Build history of the part. All positions in model axes, mm. Face numbers are marked on the shaded views. A direction names the side the tool comes from. Coordinates: 2 decimals unless noted, no trailing zeros. Loops run counter-clockwise (first coordinate to the right, second up) from the corner with the lowest first, then second, coordinate; pieces in that order, holes last. Notation, with made-up numbers: (20, 67) - (35, 67) arc R25 ccw to (35, 92) - close; hole circle Ø3 at (-9.5, -22). An arc over 180 degrees is marked (long way). One line per item, written item: value.
Autodesk Inventor part; units mm, degrees
ref_plane "YZ Plane" through (0, 0, 0) normal (1, 0, 0) x (0, 1, 0)
ref_plane "XZ Plane" through (0, 0, 0) normal (0, 1, 0) x (-1, 0, 0)
ref_plane "XY Plane" through (0, 0, 0) normal (0, 0, 1) x (1, 0, 0)
sketch "Sketch1" plane through (0, 0, 0) normal (0, 1, 0) x (-1, 0, 0)
  circle A0 centre (0, 0) radius 3.2
  dimension "d0" = 6.4
extrude "Extrusion1" add sketch "Sketch1" against normal blind 42
sketch "Sketch2" plane through (0, -42, 0) normal (0, -1, 0) x (1, 0, 0)
  circle A0 centre (0, 0) radius 6.5
  dimension "d3" = 13
extrude "Extrusion2" add sketch "Sketch2" against normal blind 20
sketch "Sketch3" plane through (0, 0, 0) normal (0, 1, 0) x (1, 0, 0)
  circle A0 centre (0, 0) radius 3.2
  line L0 (0, -3.2) -> (0, 3.2) construction
  circle A1 centre (0, -1.2) radius 0.5
  circle A2 centre (0, 1.4) radius 0.5
  dimension "d6" = 0
  dimension "d7" = 1
  dimension "d8" = 1
  dimension "d9" = 1.8
  dimension "d10" = 2.6
extrude "Extrusion3" add sketch "Sketch3" along normal blind 6 contours A1 | A2
fillet "Fillet1" radius 0.5 2 edges at (-0.5, 6, -1.4) (-0.5, 6, 1.2)
properties part number "Arc Water Sensor"
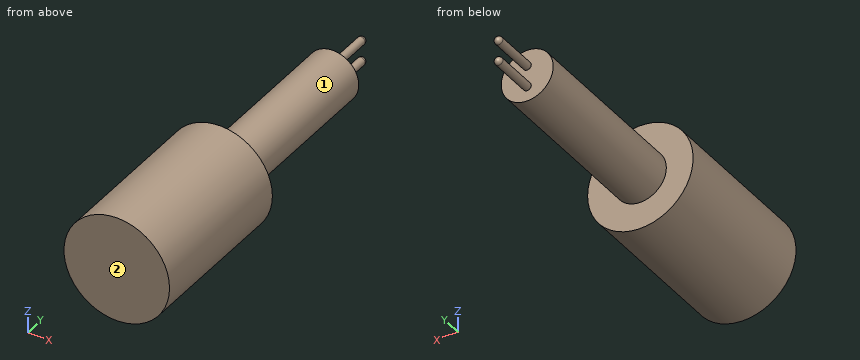
Item 1: Probe probe 1 along Y at (x, z) = (3.5, -0.25); probe 2 along Y at (x, z) = (-2.75, -0.5); probe 3 along Z at (x, y) = (-0.25, -15). List the from-to ranges inside material, lowest first. Write a range as from..to.
Check result:
probe 1: y = -42..-22
probe 2: y = -42..0
probe 3: z = -3.19..3.19
Item 2: Cut at C-C, the plane y = -11.5. Write the cut outline in (x, z).
Check result:
outline: circle Ø6.4 at (0, 0)
Item 3: Cut at B-B, the plane z = -1.4. Write the cut outline in (x, y).
Check result:
outline: (-6.35, -42) - (6.35, -42) - (6.35, -22) - (2.88, -22) - (2.88, 0) - (0.5, 0) - (0.5, 5.5) arc R0.5 ccw to (-0.5, 5.5) - (-0.5, 0) - (-2.88, 0) - (-2.88, -22) - (-6.35, -22) - close
Item 4: Cut at A-A, the plane x = 0. Write the cut outline in (y, z).
Check result:
outline: (-42, -6.5) - (-22, -6.5) - (-22, -3.2) - (0, -3.2) - (0, -1.9) - (5.5, -1.9) arc R0.5 ccw to (5.5, -0.9) - (0, -0.9) - (0, 0.7) - (5.5, 0.7) arc R0.5 ccw to (5.5, 1.7) - (0, 1.7) - (0, 3.2) - (-22, 3.2) - (-22, 6.5) - (-42, 6.5) - close
Item 5: Drop flat-ended pins along their axis: P1, Ø1, axis at x = 1.5, y = -21, coming from the -Z side; P2, Ø5, axis at x = -5, y = -12.5, coming from the -Z side; P3, Ø6, axis at x = 4, z = -3.5, coming from the +Y side. Give the stop position or say it passes through.
Check result:
P1: stops at z = -3.04
P2: stops at z = -2
P3: stops at y = 0
Item 6: Tool access for the marked faces 1 and 2: list every direction of +Z, -Z, +X, -X, +Y, -Y with a clear straight run to the whole face (end or side of a thin tool).
Check result:
face 1: +Y
face 2: +Z, -Z, +X, -X, -Y
Item 7: Cut at D-D, the plane x = 2.25. Write the cut outline in (y, z), then the cut area to 3 significant figures.
Check result:
outline: (-42, -6.1) - (-22, -6.1) - (-22, -2.28) - (0, -2.28) - (0, 2.28) - (-22, 2.28) - (-22, 6.1) - (-42, 6.1) - close
area: 344 mm^2
